from build123d import *

# Parameters (mm, degrees)
SKETCH1_W               = 19.05
SKETCH1_H               = 19.05
SKETCH1_R               = 4.826
BOSS_EXTRUDE1_DEPTH     = 12.446
CUT_EXTRUDE1_DEPTH      = 30.676723471
CUT_EXTRUDE1_DEPTH_BACK = 30.676723471


with BuildPart() as part:
    # Sketch1 → Boss-Extrude1 (new body)
    with BuildSketch(Plane.XY):
        with Locations((9.525, -9.525)):
            Rectangle(SKETCH1_W, SKETCH1_H)
        with Locations((9.525, -9.525)):
            Circle(SKETCH1_R, mode=Mode.SUBTRACT)
    extrude(amount=-BOSS_EXTRUDE1_DEPTH)

    # Sketch2 → Cut-Extrude1 (cut, two sides: drawn at the far end of the back side and taken through both)
    with BuildSketch(Plane(origin=(0, 0, 0), x_dir=(1, 0, 0), z_dir=(0, 1, 0)).offset(-CUT_EXTRUDE1_DEPTH_BACK)):
        Polygon((-35.652150586, -32.211964891), (0, 4.572), (1.6002, 6.223), (0, 7.874), (-35.652150586, 44.657964891), (-138.104791636, 44.657964891), (-138.104791636, -32.211964891), align=None)
    extrude(amount=CUT_EXTRUDE1_DEPTH + CUT_EXTRUDE1_DEPTH_BACK, mode=Mode.SUBTRACT)


solid = part.part
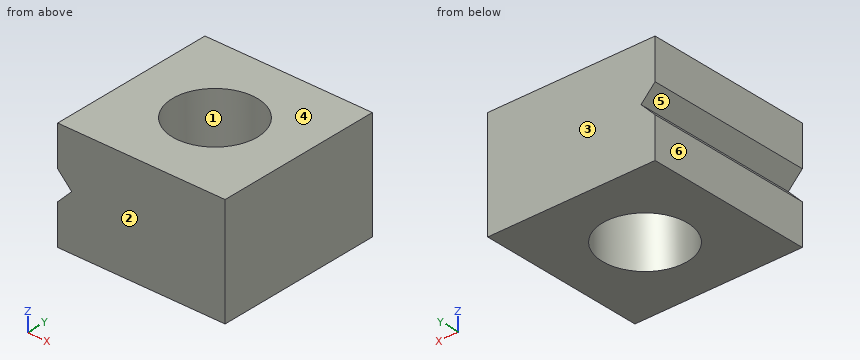
Source: CAD feature listing. Evaluate the final solid. Frame: model axes, mm. Face numbers are marked on the shaded views. A direction names the side the tool comes from. Give positions to 0.01 mm unless a question says otherwise; leave off trailing zeros. Loops run counter-clockwise (first coordinate to the right, second up) from the corner with the lowest first, then second, coordinate; pieces in that order, holes last. Notation, with made-up numbers: (53, 40.25) -> (67, 40.25) arc R27 cw to (67, 56.25) -> close; hole circle Ø3 at (4, 1.5). An arc over 180 degrees is marked (long way). Use a Markdown table: item, result. Add a question column.
1) Section query D-D, the plane y = -9. Return the cut outline in (x, z).
2) Section query C-C, the plane z = -9.25. Return the cut outline in (x, y) (3 decimals).
3) Section query B-B, the plane x = 5.5. Return the cut outline in (y, z), then the cut area to 3 significant figures.
4) Reachability of the marked faces 5 and 6 from +Z, -Z, +X, -X, +Y, -Y: full face, straight path, thin tool, end or side. Return the list, or none.
5) Pull-direction query (Y, two-part tool) for the marked faces 1, 2, 3 and 4; classes: +Y half, -Y half, draft (parallel to the pull), parting line (faces both ways), or undercut.
6) Line query: line 1 along Y through (x, z) = (8.5, -11.25); line 2 along Z through (x, y) = (1, -10.5); line 3 along X through (y, z) = (-7, -11.5). Output: solid intervals per line, ascending. Write a range as [from, to].
7) Section query A-A, the plane y = -11.75. Return the cut outline in (x, z).
Numbers:
| question | item | result |
|---|---|---|
| 1 | outline | (0, -12.45) -> (4.73, -12.45) -> (4.73, 0) -> (0, 0) -> (0, -4.57) -> (1.6, -6.22) -> (0, -7.87) -> close; (14.32, -12.45) -> (19.05, -12.45) -> (19.05, 0) -> (14.32, 0) -> close |
| 2 | outline | (0, -19.05) -> (19.05, -19.05) -> (19.05, 0) -> (0, 0) -> close; hole circle Ø9.652 at (9.525, -9.525) |
| 3 | outline | (-19.05, -12.45) -> (-12.19, -12.45) -> (-12.19, 0) -> (-19.05, 0) -> close; (-6.86, -12.45) -> (0, -12.45) -> (0, 0) -> (-6.86, 0) -> close |
| 3 | area | 171 mm2 |
| 4 | face 5 | -X, +Y, -Y |
| 4 | face 6 | +Z, -Z, -X, +Y, -Y |
| 5 | face 1 | undercut |
| 5 | face 2 | -Y half |
| 5 | face 3 | +Y half |
| 5 | face 4 | draft |
| 6 | line 1 | y = [-19.05, -14.24], [-4.81, 0] |
| 6 | line 2 | z = [-12.45, -6.84], [-5.6, 0] |
| 6 | line 3 | x = [0, 5.41], [13.64, 19.05] |
| 7 | outline | (0, -12.45) -> (5.24, -12.45) -> (5.24, 0) -> (0, 0) -> (0, -4.57) -> (1.6, -6.22) -> (0, -7.87) -> close; (13.81, -12.45) -> (19.05, -12.45) -> (19.05, 0) -> (13.81, 0) -> close |
